from build123d import *

# Parameters (mm, degrees)
F0_W      = 44
F0_H      = 65
F1_DEPTH  = 20
F2_W      = 41
F2_H      = 62
F3_DEPTH  = 18.5
F4_W      = 2
F4_H      = 5
F5_DEPTH  = 5
F7_DEPTH  = 30
F8_W      = 2
F8_H      = 5
F9_DEPTH  = 5
F11_DEPTH = 30
F13_R     = 1.625
F14_DEPTH = 17
F15_R     = 0.8
F16_DEPTH = 17


with BuildPart() as f1:
    # F0 (on Top) → F1 (new body)
    with BuildSketch(Plane.XY):
        with Locations((-23.4515, -66.719449)):
            Rectangle(F0_W, F0_H)
    extrude(amount=F1_DEPTH)

    # F2 (on face) → F3 (cut)
    with BuildSketch(Plane.XY.offset(20)):
        with Locations((-23.4515, -66.719449)):
            Rectangle(F2_W, F2_H)
    extrude(amount=-F3_DEPTH, mode=Mode.SUBTRACT)

    # F4 (on face) → F5 (join)
    with BuildSketch(Plane.XZ.offset(35.719449)):
        with Locations((-36.9515, 12)):
            Rectangle(F4_W, F4_H)
        with Locations((-9.9515, 12)):
            Rectangle(F4_W, F4_H)
    extrude(amount=F5_DEPTH)

    # F6 (on face) → F7 (cut)
    with BuildSketch(Plane(origin=(-37.9515, 0, 0), x_dir=(0, -1, 0), z_dir=(-1, 0, 0))):
        Polygon((38.219449, 14.5), (35.719449, 9.5), (40.719449, 9.5), (40.719449, 14.5), align=None)
    extrude(amount=-F7_DEPTH, mode=Mode.SUBTRACT)

    # F8 (on face) → F9 (join)
    with BuildSketch(Plane(origin=(0, -97.719449, 0), x_dir=(-1, 0, 0), z_dir=(0, 1, 0))):
        with Locations((36.9515, 12)):
            Rectangle(F8_W, F8_H)
        with Locations((9.9515, 12)):
            Rectangle(F8_W, F8_H)
    extrude(amount=F9_DEPTH)

    # F10 (on face) → F11 (cut)
    with BuildSketch(Plane.YZ.offset(-8.9515)):
        Polygon((-95.219449, 14.5), (-97.719449, 9.5), (-92.719449, 9.5), (-92.719449, 14.5), align=None)
    extrude(amount=-F11_DEPTH, mode=Mode.SUBTRACT)

    # F13 (on face) → F14 (join)
    with BuildSketch(Plane.XY.offset(1.5)):
        with Locations((-43.6515, -36.019449)):
            Circle(F13_R)
        with Locations((-3.2515, -36.019449)):
            Circle(F13_R)
        with Locations((-3.2515, -97.419449)):
            Circle(F13_R)
        with Locations((-43.6515, -97.419449)):
            Circle(F13_R)
    extrude(amount=F14_DEPTH)

    # F15 (on face) → F16 (cut)
    with BuildSketch(Plane.XY.offset(20)):
        with Locations((-43.9515, -97.719449)):
            Circle(F15_R)
        with Locations((-2.9515, -97.719449)):
            Circle(F15_R)
        with Locations((-43.9515, -35.719449)):
            Circle(F15_R)
        with Locations((-2.9515, -35.719449)):
            Circle(F15_R)
    extrude(amount=-F16_DEPTH, mode=Mode.SUBTRACT)


solid = f1.part
Check sheet for the modelled part. Datum: model origin and axes. Units: mm. A direction names the side the tool comes from. Round coordinates to 2 decimals unless told otherwise and drop trailing zeros. Order: outer loops, then holes, each group sorted by start corner. A loop starts at its lowest first (then second) coordinate and runs counter-clockwise, first axis right, second up.
Q1. Cross-section at A-A, the plane y = -73.5. Enter the section's corners in (x, z), plus the area to 4 significant figures.
Filled sheet:
outline: (-45.45, 0) - (-1.45, 0) - (-1.45, 20) - (-2.95, 20) - (-2.95, 1.5) - (-43.95, 1.5) - (-43.95, 20) - (-45.45, 20) - close
area: 121.5 mm2
Q2. Cross-section at D-D, the plane x = -10. Enter the section's corners in (y, z), plus the area to 4 significant figures.
Filled sheet:
outline: (-99.22, 0) - (-34.22, 0) - (-34.22, 20) - (-35.72, 20) - (-35.72, 14.5) - (-38.22, 14.5) - (-35.72, 9.5) - (-35.72, 1.5) - (-97.72, 1.5) - (-97.72, 9.5) - (-95.22, 14.5) - (-97.72, 14.5) - (-97.72, 20) - (-99.22, 20) - close
area: 165.5 mm2
Q3. Cross-section at C-C, the plane x = -28. Enter the section's corners in (y, z), plus the area to 3 significant figures.
Filled sheet:
outline: (-99.22, 0) - (-34.22, 0) - (-34.22, 20) - (-35.72, 20) - (-35.72, 1.5) - (-97.72, 1.5) - (-97.72, 20) - (-99.22, 20) - close
area: 153 mm2
Q4. Set-up check for faces 5 (the face through (-4, -37, 18.5)), 6 (the face through (-1.451, -67, 10)), 7 (the face through (-9.94, -96.45, 12.04)): record each of +Z, -Z, +X, -X, +Y, -Y from which the full face is reachable in a straight line by a thin tool's end or side.
Filled sheet:
face 5: +Z
face 6: +Z, -Z, +X, +Y, -Y
face 7: none
Q5. Cross-section at B-B, the plane z = 13.5. Give the number of separate pieces and of enclosed holes in the cut face, plus the area to 3 significant figures.
Filled sheet:
separate pieces: 1
enclosed holes: 5
area: 338 mm2
Q6. Scan lines: L1, parallel to X at y = -93, z = 1.75; L2, parallel to Y at x = -25, z = 8; L3, parallel to Y at x = -3.5, z = 4. Record each from-to range of solid material in increasing order.
Filled sheet:
L1: x = -45.45 to -43.95, -2.95 to -1.45
L2: y = -99.22 to -97.72, -35.72 to -34.22
L3: y = -99.22 to -98.3, -97.14 to -95.81, -37.63 to -36.3, -35.14 to -34.22
Q7. Draft check along Z on faces 1 (the face through (-24, -66, 0)), 2 (the face through (-10, -37, 14.5)), 3 (the face through (-35.952, -36, 13)), 4 (the face through (-9.97, -36.99, 12.04)). Enter one of: pulls with the +Z half, pulls with the -Z half, needs draft (parallel to the pull), parting line crosses it, or undercut.
Filled sheet:
face 1: pulls with the -Z half
face 2: pulls with the +Z half
face 3: needs draft
face 4: undercut
Q8. Depth check by flat-ended pin: P1, Ø0.6, axis at x = -43, y = -97, coming from the +Z side; P2, Ø0.6, axis at x = -10, y = -37, coming from the +Z side; P3, Ø1.5, axis at x = -36.5, y = -88.5, coming from the +Z side. Enter the tip coordinate at first touch or a pass-through.
Filled sheet:
P1: stops at z = 18.5
P2: stops at z = 14.5
P3: stops at z = 1.5
